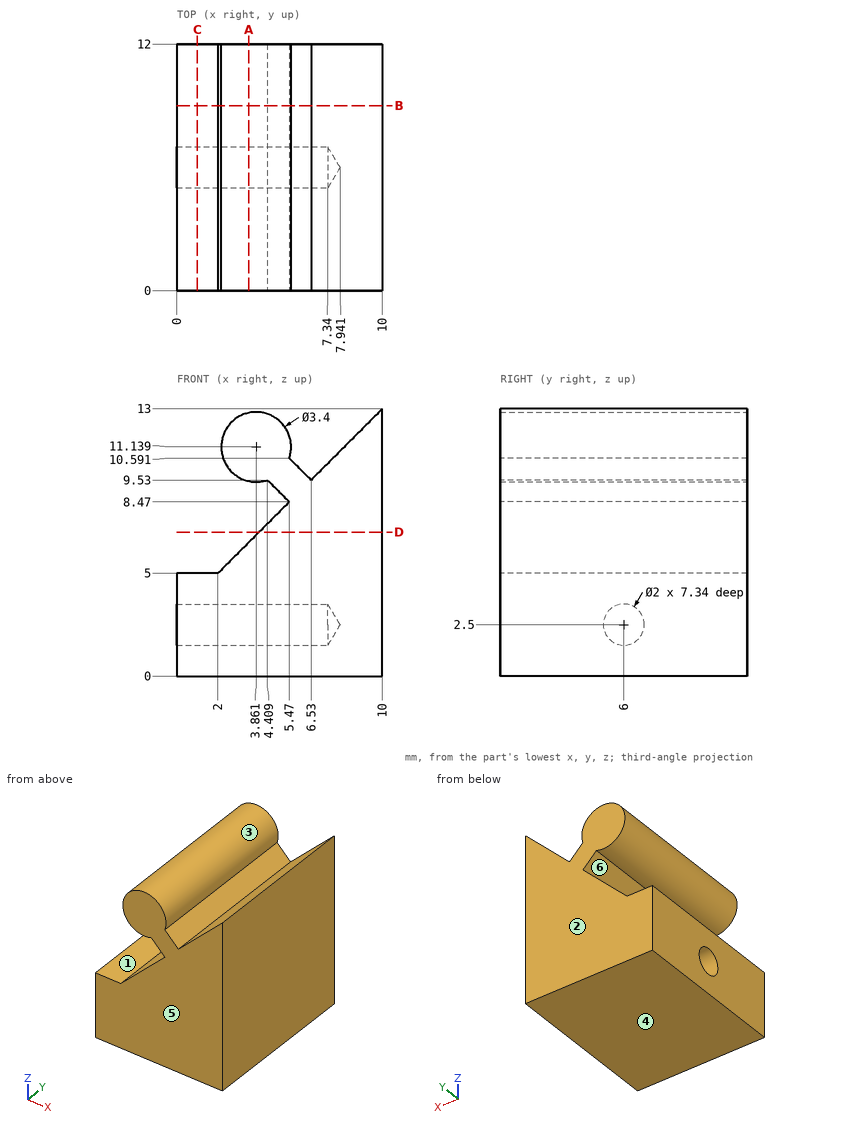
The drawing under review shows one solid part. Ordinate dimensions are in mm from its lowest x, y, z. A direction names the side the tool comes from. Round coordinates to 2 decimals unless told otherwise and drop trailing zeros. Write each loop counter-clockwise with the first axis right and the second up, starting at its lowest first coordinate (ties: lowest second). Pieces come first, ordered by that corner, then holes. Notation, with made-up numbers: (59, 28) - (96, 28) arc R10 ccw to (96, 42) - close; hole circle Ø5 at (31.25, 89.5). An arc over 180 degrees is marked (long way). Write each question's results on one line, items separated by ' | '.
Item 1: For the marked faces 1 and 2, list the 3-axis set-ups (+Z, -Z, +X, -X, +Y, -Y) from which the entire face can be reached by the end or side of a thin tool; tool diameter is ignored.
Calculated:
face 1: +Z, -X, +Y, -Y | face 2: +Z, -Z, +X, -X, +Y
Item 2: Take a section at A-A on x = 3.5. State the section outline as (y, z) points, then the cut area to 3 significant figures.
Calculated:
outline: (0, 0) - (12, 0) - (12, 6.5) - (0, 6.5) - close; (0, 9.48) - (12, 9.48) - (12, 12.8) - (0, 12.8) - close; hole circle Ø2 at (6, 2.5) | area: 115 mm^2
Item 3: For pin 1 (5 mm diameter, centred on x = 2.5, z = 9, fed in from +Y); pin 2 (1 mm diameter, centred on x = 3.5, y = 3.5, fed in from +Z), all flat-tipped, find the tip position at first contact; note any pin that passes through.
Calculated:
pin 1: stops at y = 12 | pin 2: stops at z = 12.84
Item 4: Draft analysis for pull direction Z (two halves, no side actions). For the marked faces 3, 4, 5 and 6, state which applies: pulls with the +Z half, pulls with the -Z half, needs draft (parallel to the pull), parting line crosses it, or undercut.
Calculated:
face 3: undercut | face 4: pulls with the -Z half | face 5: needs draft | face 6: undercut
Item 5: Take a section at C-C on x = 1. State the section outline as (y, z) points.
Calculated:
outline: (0, 0) - (12, 0) - (12, 5) - (0, 5) - close; hole circle Ø2 at (6, 2.5)
Item 6: Take a section at B-B on y = 9. State the section outline as (x, z) points.
Calculated:
outline: (0, 0) - (10, 0) - (10, 13) - (6.53, 9.53) - (5.47, 10.59) arc R1.7 ccw (long way) to (4.41, 9.53) - (5.47, 8.47) - (2, 5) - (0, 5) - close
Item 7: Take a section at D-D on z = 7. State the section outline as (x, y) points, then the cut area to 3 significant figures.
Calculated:
outline: (4, 0) - (10, 0) - (10, 12) - (4, 12) - close | area: 72.0 mm^2
Item 8: To check wall thickness, follow line 1 along Z through (x, y) = (1.75, 6); line 2 along Y through (x, z) = (5, 2.5); line 3 along Z through (x, y) = (5, 6). State the ranges of each line that lie inside material, in increasing order. Write a range as from..to.
Calculated:
line 1: z = 0..1.5, 3.5..5 | line 2: y = 0..5, 7..12 | line 3: z = 0..1.5, 3.5..8, 8.94..12.4
